Part print with two shaded views. Sizes in mm from the minimum x, y, z corner. Round coordinates to 2 decimals unless told otherwise and drop trailing zeros. Loops run counter-clockwise (first coordinate to the right, second up) from the corner with the lowest first, then second, coordinate; pieces in that order, holes last. Notation, with made-up numbers: (74, 76) - (101, 76) arc R34 cw to (101, 111) - close; hole circle Ø11 at (69, 48). An arc over 180 degrees is marked (long way). Write each question's results on one line, items separated by ' | '. Start each with the question number.
(1) Cut at D-D, the plane x = 36.5. List the corners of the cut face in (y, z).
(2) Cut at C-C, the plane z = 121.5. List the corners of the cut face in (x, y).
(3) Drill centre lines: L1, parallel to X at y = 10.75, z = 97.5; L2, parallel to X at y = 5.25, z = 97.5; L3, parallel to X at y = 12.5, z = 111.5. Where is each one in solid material? Low to high.
(4) Mould opens along X. For the marked faces 1, 2 and 3 say: released by +X, released by -X, zero draft, split by the parting line, or undercut.
(5) Cut at A-A, the plane z = 97.5. List the corners of the cut face in (x, y), then the cut area to 3 significant figures.
(6) Flat gauge pins, fed straight in: P1, Ø4.5, axis at x = 97.5, z = 138.41, coming from the +Y side; P2, Ø5.5, axis at x = 96.5, z = 56.5, coming from the +Y side; P3, Ø5, axis at x = 102, y = 11.5, coming from the +Z side; P4, Ø6, axis at x = 159.5, y = 9, coming from the +Z side. Where does each tip first touch, or does it go through?
(7) Cut at B-B, the plane x = 97.5. List the corners of the cut face in (y, z), then the cut area to 3 significant figures.
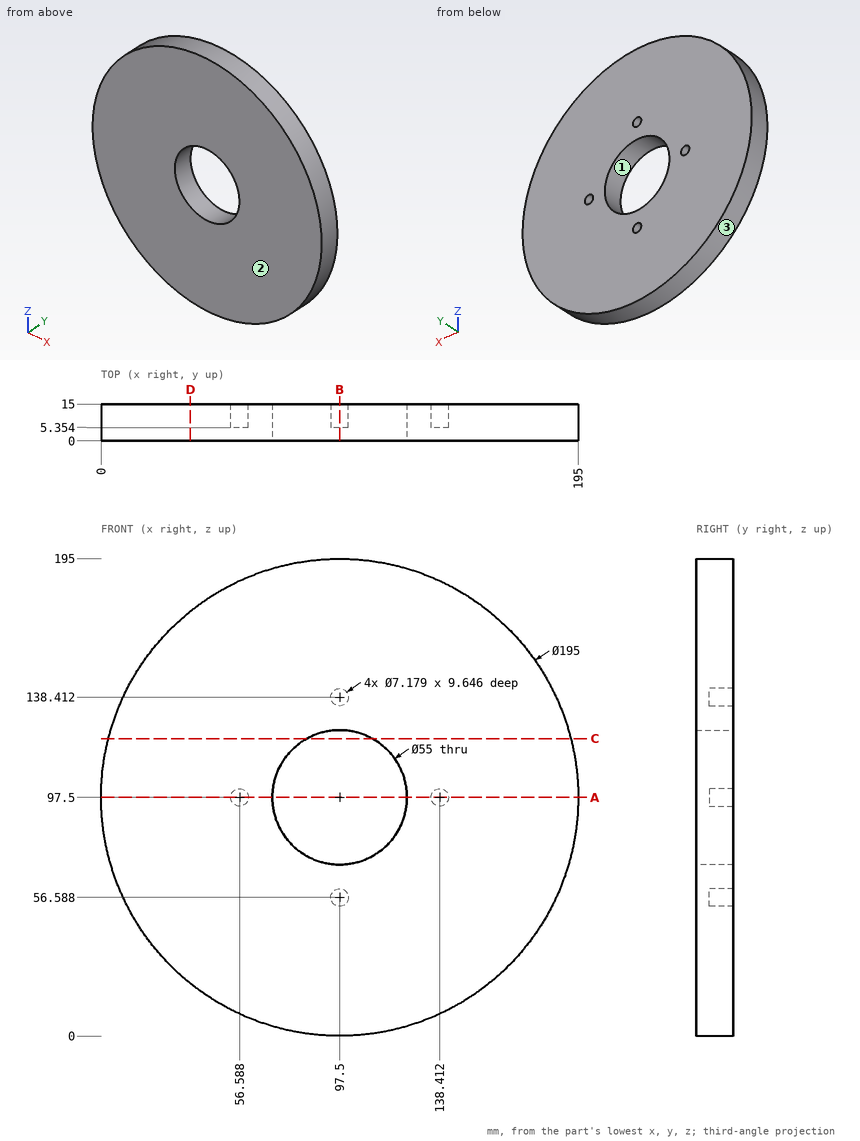
A:
1) outline: (0, 21.44) - (15, 21.44) - (15, 173.56) - (0, 173.56) - close
2) outline: (3, 0) - (84.07, 0) - (84.07, 15) - (3, 15) - close; (110.93, 0) - (192, 0) - (192, 15) - (110.93, 15) - close
3) L1: 0 to 53, 60.18 to 70, 125 to 134.82, 142 to 195 | L2: 0 to 70, 125 to 195 | L3: 1.01 to 73.83, 121.17 to 193.99
4) face 1: undercut | face 2: zero draft | face 3: split by the parting line
5) outline: (0, 0) - (70, 0) - (70, 15) - (60.18, 15) - (60.18, 5.35) - (53, 5.35) - (53, 15) - (0, 15) - close; (125, 0) - (195, 0) - (195, 15) - (142, 15) - (142, 5.35) - (134.82, 5.35) - (134.82, 15) - (125, 15) - close | area: 1,960 mm2
6) P1: y = 5.35 | P2: y = 15 | P3: z = 194.98 | P4: z = 175.12
7) outline: (0, 0) - (15, 0) - (15, 53) - (5.35, 53) - (5.35, 60.18) - (15, 60.18) - (15, 70) - (0, 70) - close; (0, 125) - (15, 125) - (15, 134.82) - (5.35, 134.82) - (5.35, 142) - (15, 142) - (15, 195) - (0, 195) - close | area: 1,960 mm2
